Source: CAD feature listing. Evaluate the final solid. Frame: model axes, mm. Face numbers are marked on the shaded views. A direction names the side the tool comes from. Give positions to 0.01 mm unless a question says otherwise; leave off trailing zeros. Order: outer loops, then holes, each group sorted by start corner. A loop starts at its lowest first (then second) coordinate and runs counter-clockwise, first axis right, second up. Notation, with made-up numbers: M 33,49.5 L 61,49.5 A30 cw 61,71.5 Z; hole C 5.25,58 d7. An arc over 180 degrees is marked long. Answer in a Markdown table with one row per item. Add a question column.
(1) Set-up query: the marked faces 1 and 2. Return all of +Z, -Z, +X, -X, +Y, -Y with unobstructed straight access to the full face (end or side cutting, diameter ignored); none if empty.
(2) Section query B-B, the plane z = 0.25. Return loops of the section in (x, y), plus the area to 3 significant figures.
(3) Material intervals for line 1 along X through (y, z) = (-4.25, -0.6); line 2 along Y through (x, z) = (-5, -1.25); line 3 along Y through (x, z) = (-14, 0.8), sorted ascending.
(4) Section query A-A, the plane y = 4. Return loops of the section in (x, z).
(5) Section query C-C, the plane y = 0. Return loops of the section in (x, z), plus the area to 3 significant figures.
(6) Section query D-D, the plane x = 10.5. Return loops of the section in (y, z), plus the area to 3 significant figures.
(7) Mould query, pull axis X, two halves, no side actions, for the marked faces 3, 4 and 5. Classes: pulls with the +X half, pulls with the -X half, needs draft (parallel to the pull), parting line crosses it, or undercut.
from build123d import *

# Parameters (mm, degrees)
CROQUIS1_R              = 0.75
SALIENTE_EXTRUIR1_DEPTH = 2.5


with BuildPart() as part:
    # Croquis1 → Saliente-Extruir1 (new, symmetric)
    with BuildSketch(Plane.XY):
        with BuildLine():
            Line((-12, 6), (12, 6))
            Line((12, 6), (12, -6))
            Line((12, -6), (17, -6))
            Line((17, -6), (17, 5.74451768))
            ThreePointArc((17, 5.74451768), (16.046491304, 8.046491304), (13.74451768, 9))
            Line((13.74451768, 9), (-13.74451768, 9))
            ThreePointArc((-13.74451768, 9), (-16.046491304, 8.046491304), (-17, 5.74451768))
            Line((-17, 5.74451768), (-17, -6))
            Line((-17, -6), (-12, -6))
            Line((-12, -6), (-12, 6))
        make_face()
        with Locations((-14, 0)):
            Circle(CROQUIS1_R, mode=Mode.SUBTRACT)
        with Locations(Location((14, 0, 0), (0, 0, 180))):
            Circle(CROQUIS1_R, mode=Mode.SUBTRACT)
    extrude(amount=SALIENTE_EXTRUIR1_DEPTH, both=True)


solid = part.part
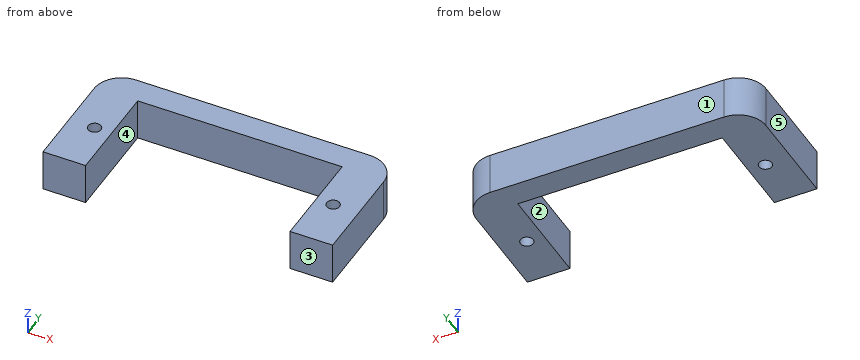
Values follow:
| question | item | result |
|---|---|---|
| 1 | face 1 | +Z, -Z, +X, -X, +Y |
| 1 | face 2 | +Z, -Z, -Y |
| 2 | outline | M -17,-6 L -12,-6 L -12,6 L 12,6 L 12,-6 L 17,-6 L 17,5.74 A3.26 ccw 13.74,9 L -13.74,9 A3.26 ccw -17,5.74 Z; hole C -14,0 d1.5; hole C 14,0 d1.5 |
| 2 | area | 214 mm² |
| 3 | line 1 | x = -17 to -12, 12 to 17 |
| 3 | line 2 | y = 6 to 9 |
| 3 | line 3 | y = -6 to -0.75, 0.75 to 8.99 |
| 4 | outline | M -17,-2.5 L -12,-2.5 L -12,2.5 L -17,2.5 Z; M 12,-2.5 L 17,-2.5 L 17,2.5 L 12,2.5 Z |
| 5 | outline | M -17,-2.5 L -14.75,-2.5 L -14.75,2.5 L -17,2.5 Z; M -13.25,-2.5 L -12,-2.5 L -12,2.5 L -13.25,2.5 Z; M 12,-2.5 L 13.25,-2.5 L 13.25,2.5 L 12,2.5 Z; M 14.75,-2.5 L 17,-2.5 L 17,2.5 L 14.75,2.5 Z |
| 5 | area | 35.0 mm² |
| 6 | outline | M 6,-2.5 L 9,-2.5 L 9,2.5 L 6,2.5 Z |
| 6 | area | 15.0 mm² |
| 7 | face 3 | needs draft |
| 7 | face 4 | undercut |
| 7 | face 5 | pulls with the -X half |
